from build123d import *
from build123d.topology import SkipClean

# Parameters (mm, degrees)
SKETCH1_R            = 150
BOSS_EXTRUDE1_DEPTH  = 200
BOSS_EXTRUDE11_DEPTH = 300
BOSS_EXTRUDE14_START = -300
SKETCH12_R           = 125
BOSS_EXTRUDE14_DEPTH = 400
SKETCH13_W           = 400
SKETCH13_H           = 350
SKETCH13_R           = 10
BOSS_EXTRUDE15_DEPTH = 50
SKETCH13_3_W         = 50
SKETCH13_3_H         = 80
SKETCH13_3_R         = 10
BOSS_EXTRUDE16_DEPTH = 20
BOSS_EXTRUDE17_DEPTH = 90
SKETCH16_R           = 20
BOSS_EXTRUDE18_DEPTH = 150
FILLET2_R            = 10
FILLET3_R            = 20


with BuildPart() as part:
    # Sketch1 → Boss-Extrude1 (new body)
    with BuildSketch(Plane.XY):
        Circle(SKETCH1_R)
    extrude(amount=BOSS_EXTRUDE1_DEPTH)

    # Sketch7 → Boss-Extrude11 (add)
    with SkipClean():  # the faces are left unmerged after this step: merging them gives an invalid solid
        with BuildSketch(Plane.XY.offset(200)):
            with BuildLine():
                Line((-90, 120), (90, 120))
                ThreePointArc((90, 120), (101.396020382, 110.538893837), (111.803398875, 100))
                Line((111.803398875, 100), (-111.803398875, 100))
                ThreePointArc((-111.803398875, 100), (-101.396020382, 110.538893837), (-90, 120))
            make_face()
            with BuildLine():
                Line((-126.885775404, 80), (126.885775404, 80))
                ThreePointArc((126.885775404, 80), (132.559251115, 70.200035213), (137.477270849, 60))
                Line((137.477270849, 60), (-137.477270849, 60))
                ThreePointArc((-137.477270849, 60), (-132.559251115, 70.200035213), (-126.885775404, 80))
            make_face()
            with BuildLine():
                Line((144.16342013, -41.435592144), (-144.16342013, -41.435592144))
                ThreePointArc((-144.16342013, -41.435592144), (-146.803816882, -30.799989431), (-148.660687473, -20))
                Line((-148.660687473, -20), (148.660687473, -20))
                ThreePointArc((148.660687473, -20), (146.803816882, -30.799989431), (144.16342013, -41.435592144))
            make_face()
            with BuildLine():
                Line((111.803398875, -100), (-111.803398875, -100))
                ThreePointArc((-111.803398875, -100), (-101.396020382, -110.538893837), (-90, -120))
                Line((-90, -120), (90, -120))
                ThreePointArc((90, -120), (101.396020382, -110.538893837), (111.803398875, -100))
            make_face()
            with BuildLine():
                Line((144.568322948, 40), (-144.568322948, 40))
                ThreePointArc((-144.568322948, 40), (-146.955139883, 30.069700063), (-148.660687473, 20))
                Line((-148.660687473, 20), (148.660687473, 20))
                ThreePointArc((148.660687473, 20), (146.955139883, 30.069700063), (144.568322948, 40))
            make_face()
            with BuildLine():
                Line((137.477270849, -60), (-137.477270849, -60))
                ThreePointArc((-137.477270849, -60), (-133.599215205, -68.20007109), (-129.232599216, -76.150740639))
                Line((-129.232599216, -76.150740639), (129.232599216, -76.150740639))
                ThreePointArc((129.232599216, -76.150740639), (133.599215205, -68.20007109), (137.477270849, -60))
            make_face()
        extrude(amount=BOSS_EXTRUDE11_DEPTH)



with BuildPart() as body_2:
    # Sketch12 → Boss-Extrude14 (new body)
    with BuildSketch(Plane.XY.offset(500).offset(BOSS_EXTRUDE14_START)):
        Circle(SKETCH12_R)
    extrude(amount=BOSS_EXTRUDE14_DEPTH)


with BuildPart() as body_3:
    # Sketch13 → Boss-Extrude15 (new body)
    with BuildSketch(Plane(origin=(0, -210, 0), x_dir=(-1, 0, 0), z_dir=(0, -1, 0))):
        with Locations((0, -274.735715433)):
            Rectangle(SKETCH13_W, SKETCH13_H)
        with Locations(Location((-175, -139.735715433, 0), (0, 0, 180))):
            Circle(SKETCH13_R, mode=Mode.SUBTRACT)
        with Locations(Location((175, -139.735715433, 0), (0, 0, 180))):
            Circle(SKETCH13_R, mode=Mode.SUBTRACT)
        with Locations(Location((175, -409.735715433, 0), (0, 0, 180))):
            Circle(SKETCH13_R, mode=Mode.SUBTRACT)
        with Locations(Location((-175, -409.735715433, 0), (0, 0, 180))):
            Circle(SKETCH13_R, mode=Mode.SUBTRACT)
    extrude(amount=-BOSS_EXTRUDE15_DEPTH)

    # Sketch13<3> → Boss-Extrude16 (add)
    # profile 1 of 4: a face of its own
    with BuildSketch(Plane(origin=(0, -210, 0), x_dir=(-1, 0, 0), z_dir=(0, -1, 0))):
        with Locations((-175, -409.735715433)):
            Rectangle(SKETCH13_3_W, SKETCH13_3_H)
        with Locations(Location((-175, -409.735715433, 0), (0, 0, 180))):
            Circle(SKETCH13_3_R, mode=Mode.SUBTRACT)
    # profile 2 of 4: a face of its own
    with BuildSketch(Plane(origin=(0, -210, 0), x_dir=(-1, 0, 0), z_dir=(0, -1, 0))):
        with Locations((-175, -139.735715433)):
            Rectangle(SKETCH13_3_W, SKETCH13_3_H)
        with Locations(Location((-175, -139.735715433, 0), (0, 0, 180))):
            Circle(SKETCH13_3_R, mode=Mode.SUBTRACT)
    # profile 3 of 4: a face of its own
    with BuildSketch(Plane(origin=(0, -210, 0), x_dir=(-1, 0, 0), z_dir=(0, -1, 0))):
        with Locations((175, -409.735715433)):
            Rectangle(SKETCH13_3_W, SKETCH13_3_H)
        with Locations(Location((175, -409.735715433, 0), (0, 0, 180))):
            Circle(SKETCH13_3_R, mode=Mode.SUBTRACT)
    # profile 4 of 4: a face of its own
    with BuildSketch(Plane(origin=(0, -210, 0), x_dir=(-1, 0, 0), z_dir=(0, -1, 0))):
        with Locations((175, -139.735715433)):
            Rectangle(SKETCH13_3_W, SKETCH13_3_H)
        with Locations(Location((175, -139.735715433, 0), (0, 0, 180))):
            Circle(SKETCH13_3_R, mode=Mode.SUBTRACT)
    extrude(amount=BOSS_EXTRUDE16_DEPTH)


with BuildPart() as part_1:
    with SkipClean():  # the faces are left unmerged after this step: merging them gives an invalid solid
        add(part.part)

        add(body_2.part)  # Boss-Extrude17 merges body 2

        add(body_3.part)  # Boss-Extrude17 merges body 3
        # Sketch14 → Boss-Extrude17 (add, symmetric)
        with BuildSketch(Plane.XY.offset(274.735715433)):
            Polygon((-200, -160), (200, -160), (100, -100), (-100, -100), align=None)
        extrude(amount=BOSS_EXTRUDE17_DEPTH, both=True)

    # Sketch16 → Boss-Extrude18 (add)
    with BuildSketch(Plane.XY.offset(600)):
        Circle(SKETCH16_R)
    extrude(amount=BOSS_EXTRUDE18_DEPTH)

    # Fillet2
    fillet2_edges = [part_1.edges().sort_by_distance(p)[0] for p in [
        (-20, 0, 600),
    ]]
    fillet(fillet2_edges, radius=FILLET2_R)

    # Fillet3
    fillet3_edges = [part_1.edges().sort_by_distance(p)[0] for p in [
        (-125, 0, 600),
        (-150, 0, 0),
    ]]
    fillet(fillet3_edges, radius=FILLET3_R)


solid = part_1.part
For this review, take the finished solid that the model builds, in its own axes (mm). A direction names the side the tool comes from. Round coordinates to 2 decimals unless told otherwise and drop trailing zeros. Write each loop counter-clockwise with the first axis right and the second up, starting at its lowest first coordinate (ties: lowest second). Pieces come first, ordered by that corner, then holes. Notation, with made-up numbers: (-34.75, 73.5) -> (4.25, 73.5) arc R12 cw to (4.25, 96.5) -> close; hole circle Ø3 at (-9.5, 86). An arc over 180 degrees is marked (long way). Use CSV: the item, a comma, the result in double quotes.
(1) Consider section A-A, the plane x = -175. Give the boundary of the cut face in (y, z), plus the area to 3 significant figures.
Computed values:
outline,"(-230, 99.74) -> (-160, 99.74) -> (-160, 129.74) -> (-230, 129.74) -> close; (-230, 149.74) -> (-160, 149.74) -> (-160, 184.74) -> (-145, 184.74) -> (-145, 364.74) -> (-160, 364.74) -> (-160, 399.74) -> (-230, 399.74) -> (-230, 369.74) -> (-210, 369.74) -> (-210, 179.74) -> (-230, 179.74) -> close; (-230, 419.74) -> (-160, 419.74) -> (-160, 449.74) -> (-230, 449.74) -> close"
area,"20,600 mm²"
(2) Consider section B-B, the plane y = 0. Give the boundary of the cut face in (x, z), plus the area to 3 significant figures.
Computed values:
outline,"(-150, 20) arc R20 ccw to (-130, 0) -> (130, 0) arc R20 ccw to (150, 20) -> (150, 200) -> (125, 200) -> (125, 580) arc R20 ccw to (105, 600) -> (30, 600) arc R10 cw to (20, 610) -> (20, 750) -> (-20, 750) -> (-20, 610) arc R10 cw to (-30, 600) -> (-105, 600) arc R20 ccw to (-125, 580) -> (-125, 200) -> (-150, 200) -> close"
area,"166,000 mm²"
(3) Consider section C-C, the plane x = 0. Give the boundary of the cut face in (y, z).
Computed values:
outline,"(-210, 99.74) -> (-160, 99.74) -> (-160, 184.74) -> (-150, 184.74) -> (-150, 20) arc R20 ccw to (-130, 0) -> (130, 0) arc R20 ccw to (150, 20) -> (150, 200) -> (125, 200) -> (125, 580) arc R20 ccw to (105, 600) -> (30, 600) arc R10 cw to (20, 610) -> (20, 750) -> (-20, 750) -> (-20, 610) arc R10 cw to (-30, 600) -> (-105, 600) arc R20 ccw to (-125, 580) -> (-125, 364.74) -> (-160, 364.74) -> (-160, 449.74) -> (-210, 449.74) -> close"
(4) To check wall thickness, follow L1, parallel to Z at x = -175, y = -219.25; L2, parallel to Z at x = -175, y = -194; L3, parallel to Z at x = 178, y = -164.5. State the ranges of each line that lie inside material, in increasing order. Write a range as [from, to].
Computed values:
L1,"[99.74, 129.74], [149.74, 179.74], [369.74, 399.74], [419.74, 449.74]"
L2,"[99.74, 129.74], [149.74, 399.74], [419.74, 449.74]"
L3,"[99.74, 130.2], [149.28, 400.2], [419.28, 449.74]"
(5) Clearance check with flat-ended pins moving along their axes: P1, Ø2, axis at x = -112.5, z = 530, coming from the +Y side; P2, Ø18, axis at x = 116.5, y = -71.5, coming from the +Z side; P3, Ø3, axis at x = 16, y = -137, coming from the -Z side. State where each tip first meets the part, or that it passes through.
Computed values:
P1,"y = 56.5"
P2,"z = 500"
P3,"z = 1.06"
(6) For faces 1 (the face through (154.43, -132.66, 276)), 2 (the face through (-4.336, -19.524, 679.02)), 3 (the face through (82, 110, 500)), 4 (the face through (150, -220, 410)), list the 3-axis set-ups (+Z, -Z, +X, -X, +Y, -Y) from which the entire face can be reached by the end or side of a thin tool; tool diameter is ignored.
Computed values:
face 1,"+Z, -Z, +X"
face 2,"+Z"
face 3,"+Z, +X, +Y"
face 4,"+Z, -Z, -Y"
(7) Draft analysis for pull direction Y (two halves, no side actions). For faces 5 (the face through (-127, -51, 200)), 6 (the face through (-81, 110, 500)), 7 (the face through (-169, -230, 130)), state which applies: +Y half, -Y half, draft (parallel to the pull), parting line (faces both ways), or undercut.
Computed values:
face 5,"undercut"
face 6,"draft"
face 7,"-Y half"
